from build123d import *

# Parameters (mm, degrees)
SKETCH1_R           = 8.5
BOSS_EXTRUDE1_DEPTH = 4.4
SKETCH3_R           = 5.8
CUT_EXTRUDE1_DEPTH  = 4
BOSS_EXTRUDE3_START = 3
SKETCH4_R           = 8.5
SKETCH4_R_2         = 7.5
BOSS_EXTRUDE3_DEPTH = 3
BOSS_EXTRUDE4_DEPTH = 0.6


with BuildPart() as part:
    # Sketch1 → Boss-Extrude1 (new body)
    with BuildSketch(Plane.XY):
        Circle(SKETCH1_R)
    extrude(amount=BOSS_EXTRUDE1_DEPTH)

    # Sketch3 → Cut-Extrude1 (cut)
    with BuildSketch(Plane(origin=(0, 0, 0), x_dir=(-1, 0, 0), z_dir=(0, 0, -1))):
        Circle(SKETCH3_R)
    extrude(amount=-CUT_EXTRUDE1_DEPTH, mode=Mode.SUBTRACT)

    # Sketch4 → Boss-Extrude3 (add)
    with BuildSketch(Plane(origin=(0, 0, 0), x_dir=(-1, 0, 0), z_dir=(0, 0, -1)).offset(BOSS_EXTRUDE3_START)):
        Circle(SKETCH4_R)
        Circle(SKETCH4_R_2, mode=Mode.SUBTRACT)
    extrude(amount=-BOSS_EXTRUDE3_DEPTH)

    # Sketch6 → Cut-Revolve1 (revolve, cut)
    with BuildSketch(Plane(origin=(0, 0, 0), x_dir=(1, 0, 0), z_dir=(0, 1, 0)), mode=Mode.PRIVATE) as cut_revolve1_sk:
        Polygon((7.5, 0), (5.8, -1.7), (5.8, 0), align=None)
    revolve(cut_revolve1_sk.sketch.rotate(Axis((0, 0, -5.5), (0, 0, 1)), 180), axis=Axis((0, 0, -5.5), (0, 0, 1)), mode=Mode.SUBTRACT)

    # Sketch2 → Boss-Extrude4 (add)
    with BuildSketch(Plane.XY.offset(4.4)):
        Polygon((-5.631532004, 2.878926263), (-2.811019183, 5.699439083), (-2.811019183, 3.443028827), (5.368467996, 3.443028827), (5.368467996, 2.314823699), (-2.811019183, 2.314823699), (-2.811019183, 0.199439083), align=None)
        Polygon((5.368467996, -2.480048096), (2.547955176, -5.300560917), (2.547955176, -3.04415066), (-5.631532004, -3.04415066), (-5.631532004, -1.915945532), (2.547955176, -1.915945532), (2.547955176, 0.199439083), align=None)
    extrude(amount=BOSS_EXTRUDE4_DEPTH)


solid = part.part
Could you check a few things on this model? Use its own coordinates, in mm. A direction names the side the tool comes from. Coordinates: 2 decimals unless noted, no trailing zeros. Order: outer loops, then holes, each group sorted by start corner. A loop starts at its lowest first (then second) coordinate and runs counter-clockwise, first axis right, second up. Notation, with made-up numbers: (-20.75, 56.5) - (36.25, 56.5) arc R10 ccw to (36.25, 61.5) - close; hole circle Ø3 at (53, 4.5). An arc over 180 degrees is marked (long way). Answer in a Markdown table with one row per item. Add a question column.
(1) If we mould it in two halves opening along Y, with no side actions, what happens to faces 4 (the face through (-4.2, 1.52, 4.7)), 5 (the face through (-1, 3, 5)), 6 (the face through (-4.24, 4.27, 4.7)), 7 (the face through (3.938, -1.122, 4.696))? For each: released by +Y, released by -Y, zero draft, split by the parting line, or undercut.
(2) I need wall thicknesses on L1, parallel to X at y = 0, z = 2.5; L2, parallel to Y at x = 0, z = -1.7. Which ranges of each line are inside material? Lowest first, please.
(3) Will these pins go through, and if not, where does the flat tip stop? pin 1 (0.5 mm diameter, centred on y = 1.5, z = 4.5, fed in from +X); pin 2 (6 mm diameter, centred on x = 0, y = -2.5, fed in from -Z); pin 3 (0.5 mm diameter, centred on y = -2.5, z = 4.5, fed in from -X).
(4) On a 3-axis mill with a long thin cutter (end or side, diameter ignored), from which of +Z, -Z, +X, -X, +Y, -Y can I reach the whole of each face in a straight line? I mean faces 1 (the face through (0, -8, -3)), 2 (the face through (3.98, -3.87, 4.7)), 3 (the face through (5.794, 0.255, 2.834)). Say none if no direction works.
(5) If we section it at A-A, the plane x = 0: Please give me the cut outline in (y, z), then the cut area to 3 significant figures.
(6) If we section it at B-B, the plane z = -1.75: Please give me the cut outline in (x, y), then the cut area to 3 significant figures.
(7) If we section it at C-C, the plane z = 3.5: Please give me the cut outline in (x, y), then the cut area to 3 significant figures.
Results are:
| question | item | result |
|---|---|---|
| 1 | face 4 | undercut |
| 1 | face 5 | zero draft |
| 1 | face 6 | released by +Y |
| 1 | face 7 | undercut |
| 2 | L1 | x = -8.5 to -5.8, 5.8 to 8.5 |
| 2 | L2 | y = -8.5 to -7.5, 7.5 to 8.5 |
| 3 | pin 1 | stops at x = 8.4 |
| 3 | pin 2 | stops at z = 4 |
| 3 | pin 3 | stops at x = -8.19 |
| 4 | face 1 | -Z, +X, -X, +Y, -Y |
| 4 | face 2 | +Z, +X, -Y |
| 4 | face 3 | -Z |
| 5 | outline | (-8.5, -3) - (-7.5, -3) - (-7.5, 0) - (-5.8, 1.7) - (-5.8, 4) - (5.8, 4) - (5.8, 1.7) - (7.5, 0) - (7.5, -3) - (8.5, -3) - (8.5, 4.4) - (3.44, 4.4) - (3.44, 5) - (2.31, 5) - (2.31, 4.4) - (-1.92, 4.4) - (-1.92, 5) - (-3.04, 5) - (-3.04, 4.4) - (-8.5, 4.4) - close |
| 5 | area | 32.9 mm2 |
| 6 | outline | circle Ø17 at (0, 0); hole circle Ø15 at (0, 0) |
| 6 | area | 50.3 mm2 |
| 7 | outline | circle Ø17 at (0, 0); hole circle Ø11.6 at (0, 0) |
| 7 | area | 121 mm2 |
